Verification items for the finished model (mm, model axes). Face numbers are marked on the shaded views. Round coordinates to 2 decimals unless told otherwise and drop trailing zeros. Order: outer loops, then holes, each group sorted by start corner. A loop starts at its lowest first (then second) coordinate and runs counter-clockwise, first axis right, second up. Notation, with made-up numbers: (62.25, 4) -> (100.25, 4) arc R34 ccw to (100.25, 39) -> close; hole circle Ø8 at (75, -17.5). An arc over 180 degrees is marked (long way). Return JSON: item names as keys, results as strings. Group by question number.
Item 1: Draft check along X on the marked faces 1, 2 and 3. Enter one of: pulls with the +X half, pulls with the -X half, needs draft (parallel to the pull), parting line crosses it, or undercut.
Item 2: Scan lines: probe 1 along X at (y, z) = (18, -3.1); probe 2 along X at (y, z) = (-18, -2.1); probe 3 along Y at (x, z) = (-7, -2.55). Record each from-to range of solid material in increasing order. Write a range as from..to.
Item 3: Depth check by flat-ended pin: pin 1 Ø3 at (x, z) = (-13, -3) entering from -Y; pin 2 Ø3 at (x, y) = (-7, 1) entering from -Z. Enter the tip coordinate at first touch or a pass-through.
Item 4: Sectioned sample at C-C on y = 7. Record the cut outline in (x, z), plus the area to 3 significant figures.
Item 5: Sectioned sample at A-A on x = 1. Record the cut outline in (y, z).
Item 6: Sectioned sample at D-D on x = 14. Record the cut outline in (y, z).
Item 7: Sectioned sample at B-B on z = -0.9. Record the cut outline in (x, y).
```python
from build123d import *

# Parameters (mm, degrees)
SKETCH1_W           = 40
SKETCH1_H           = 40
EXTRUDE1_DEPTH      = 6
SKETCH8_R           = 6
CUT_EXTRUDE6_DEPTH  = 6
SKETCH5_R           = 1.5
CUT_EXTRUDE4_DEPTH  = 6
CIRPATTERN1_COUNT   = 3
CUT_EXTRUDE13_DEPTH = 3
SKETCH20_R          = 4
CUT_EXTRUDE14_DEPTH = 3
SKETCH25_R          = 1.25
EXTRUDE4_DEPTH      = 3
SKETCH27_R          = 1.25
EXTRUDE9_DEPTH      = 10
EXTRUDE7_START      = -10
SKETCH29_R          = 1.25
EXTRUDE7_DEPTH      = 10


# Read off the part's stored shape, not the designer's step: M3 Tapped Hole1
with BuildPart() as part:
    # Sketch1 → Extrude1 (new body)
    with BuildSketch(Plane.XY):
        with Locations((4, 0)):
            Rectangle(SKETCH1_W, SKETCH1_H)
    extrude(amount=-EXTRUDE1_DEPTH)

    # Sketch8 → Cut-Extrude6 (cut)
    with BuildSketch(Plane(origin=(0, 0, -6), x_dir=(-1, 0, 0), z_dir=(0, 0, -1))):
        with Locations((-11, 0)):
            Circle(SKETCH8_R)
    extrude(amount=-CUT_EXTRUDE6_DEPTH, mode=Mode.SUBTRACT)

    # Sketch5 → Cut-Extrude4 (cut)
    with BuildSketch(Plane(origin=(0, 0, -6), x_dir=(-1, 0, 0), z_dir=(0, 0, -1))):
        with Locations((-10, -10.95445115)):
            Circle(SKETCH5_R)
    cut_extrude4 = extrude(amount=-CUT_EXTRUDE4_DEPTH, mode=Mode.SUBTRACT)

    # CirPattern1: Cut-Extrude4 ×3 about axis
    cirpattern1_axis = Axis((11, 0, 0), (0, 0, 1))
    for i in range(1, CIRPATTERN1_COUNT):
        add(cut_extrude4.rotate(cirpattern1_axis, i * 360 / CIRPATTERN1_COUNT), mode=Mode.SUBTRACT)

    # Sketch19 → Cut-Extrude13 (cut)
    with BuildSketch(Plane(origin=(0, 0, -6), x_dir=(-1, 0, 0), z_dir=(0, 0, -1))):
        with BuildLine():
            Line((10, 4), (0, 4))
            ThreePointArc((0, 4), (-2.828427125, 2.828427125), (-4, 0))
            Line((-4, 0), (-4, -10))
            Line((-4, -10), (0, -10))
            ThreePointArc((0, -10), (7.071067812, -7.071067812), (10, 0))
            Line((10, 0), (10, 4))
        make_face()
    extrude(amount=-CUT_EXTRUDE13_DEPTH, mode=Mode.SUBTRACT)

    # Sketch20 → Cut-Extrude14 (cut)
    with BuildSketch(Plane(origin=(0, 0, -3), x_dir=(-1, 0, 0), z_dir=(0, 0, -1))):
        with Locations(Location((0, 0, 0), (0, 0, 180))):
            Circle(SKETCH20_R)
    extrude(amount=-CUT_EXTRUDE14_DEPTH, mode=Mode.SUBTRACT)

    # Sketch25 → Extrude4 (cut)
    with BuildSketch(Plane(origin=(0, 0, -3), x_dir=(-1, 0, 0), z_dir=(0, 0, -1))):
        with Locations((-1, -7)):
            Circle(SKETCH25_R)
        with Locations((7, 1)):
            Circle(SKETCH25_R)
    extrude(amount=-EXTRUDE4_DEPTH, mode=Mode.SUBTRACT)

    # Sketch27 → Extrude9 (cut)
    with BuildSketch(Plane(origin=(0, 20, 0), x_dir=(1, 0, 0), z_dir=(0, 1, 0))):
        with Locations(Location((-13, 3, 0), (0, 0, 180))):
            Circle(SKETCH27_R)
        with Locations(Location((21, 3, 0), (0, 0, 180))):
            Circle(SKETCH27_R)
    extrude(amount=-EXTRUDE9_DEPTH, mode=Mode.SUBTRACT)

    # Sketch29 → Extrude7 (cut)
    with BuildSketch(Plane.XZ.offset(20).offset(EXTRUDE7_START)):
        with Locations(Location((-13, -3, 0), (0, 0, 180))):
            Circle(SKETCH29_R)
        with Locations(Location((21, -3, 0), (0, 0, 180))):
            Circle(SKETCH29_R)
    extrude(amount=EXTRUDE7_DEPTH, mode=Mode.SUBTRACT)

    # M3 Tapped Hole1 outline → M3 Tapped Hole1 (revolve, cut)
    with BuildSketch(Plane(origin=(-13, 0, -3), x_dir=(1, 0, 0), z_dir=(0, 0, 1))):
        Polygon((1.25, -10), (0, -9.248924226), (0, -10), align=None)
        Polygon((0, 10), (0, 9.248924226), (1.25, 10), align=None)
    revolve(axis=Axis((-13, 0, -3), (0, 1, 0)), mode=Mode.SUBTRACT)

    # M3 Tapped Hole1 2 outline → M3 Tapped Hole1 2 (revolve, cut)
    with BuildSketch(Plane(origin=(21, 0, -3), x_dir=(1, 0, 0), z_dir=(0, 0, 1))):
        Polygon((1.25, -10), (0, -9.248924226), (0, -10), align=None)
        Polygon((0, 10), (0, 9.248924226), (1.25, 10), align=None)
    revolve(axis=Axis((21, 0, -3), (0, 1, 0)), mode=Mode.SUBTRACT)


solid = part.part
```
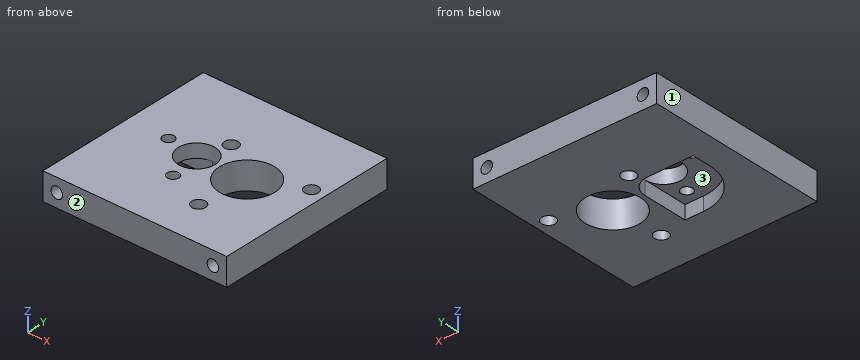
Recorded:
{
 "1": {"face 1": "pulls with the -X half", "face 2": "needs draft", "face 3": "undercut"},
 "2": {"probe 1": "-16..-14.25, -11.75..19.75, 22.25..24", "probe 2": "-16..-13.87, -12.13..20.13, 21.87..24", "probe 3": "-20..-0.25, 2.25..20"},
 "3": {"pin 1": "y = -20", "pin 2": "z = -3"},
 "4": {"outline": "(-16, -6) -> (0.66, -6) -> (0.66, 0) -> (-16, 0) -> close; (3.36, -6) -> (24, -6) -> (24, 0) -> (3.36, 0) -> close", "area": "224 mm²"},
 "5": {"outline": "(-20, -6) -> (-10, -6) -> (-10, -3) -> (-8.25, -3) -> (-8.25, 0) -> (-20, 0) -> close; (-5.75, -3) -> (-3.87, -3) -> (-3.87, 0) -> (-5.75, 0) -> close; (3.87, -6) -> (5.24, -6) -> (5.24, 0) -> (3.87, 0) -> close; (7.45, -6) -> (20, -6) -> (20, 0) -> (7.45, 0) -> close"},
 "6": {"outline": "(-20, -6) -> (-5.2, -6) -> (-5.2, 0) -> (-20, 0) -> close; (5.2, -6) -> (20, -6) -> (20, 0) -> (5.2, 0) -> close"},
 "7": {"outline": "(-16, -20) -> (24, -20) -> (24, 20) -> (-16, 20) -> close; hole circle Ø2.5 at (-7, 1); hole circle Ø8 at (0, 0); hole circle Ø2.5 at (1, -7); hole circle Ø3 at (2.01, 6.34); hole circle Ø12 at (11, 0); hole circle Ø3 at (10, -10.95); hole circle Ø3 at (20.99, 4.61)"}
}
